from build123d import *

# Parameters (mm, degrees)
ESQUISSE1_R        = 0.068980455
ESQUISSE1_R_2      = 0.06150295
ESQUISSE1_W        = 0.337022694
ESQUISSE1_H        = 5.280022209
BOSS_EXTRU_1_DEPTH = 0.1


with BuildPart() as part:
    # Esquisse1 → Boss.-Extru.1 (new body)
    with BuildSketch(Plane.XY):
        with BuildLine():
            Line((69.009405392, 230.580792913), (69.009405392, 229.722196339))
            ThreePointArc((69.009405392, 229.722196339), (68.979401433, 229.479075631), (68.891190034, 229.250544089))
            Line((68.891190034, 229.250544089), (68.752437477, 228.991137135))
            ThreePointArc((68.752437477, 228.991137135), (68.664226077, 228.762605593), (68.634222119, 228.519484885))
            Line((68.634222119, 228.519484885), (68.634222119, 222.299593089))
            ThreePointArc((68.634222119, 222.299593089), (68.467011491, 221.746003113), (68.021298395, 221.377545392))
            Line((68.021298395, 221.377545392), (63.492336438, 219.476283954))
            ThreePointArc((63.492336438, 219.476283954), (63.046623342, 219.107826233), (62.879412715, 218.554236256))
            Line((62.879412715, 218.554236256), (62.879412715, 215.999425613))
            ThreePointArc((62.879412715, 215.999425613), (62.823397918, 215.841724183), (62.680454788, 215.754691662))
            ThreePointArc((62.680454788, 215.754691662), (62.265082422, 215.243750871), (62.680454788, 214.732810081))
            ThreePointArc((62.680454788, 214.732810081), (62.823397918, 214.645777559), (62.879412715, 214.48807613))
            Line((62.879412715, 214.48807613), (62.879412715, 211.933337892))
            ThreePointArc((62.879412715, 211.933337892), (62.80618941, 211.756561196), (62.629412715, 211.683337892))
            Line((62.629412715, 211.683337892), (50.34681626, 211.683337892))
            ThreePointArc((50.34681626, 211.683337892), (50.170039564, 211.756561196), (50.09681626, 211.933337892))
            Line((50.09681626, 211.933337892), (50.09681626, 214.506095719))
            ThreePointArc((50.09681626, 214.506095719), (50.14774452, 214.657325486), (50.2797798, 214.746940302))
            ThreePointArc((50.2797798, 214.746940302), (50.65644704, 215.242767306), (50.2797798, 215.73859431))
            ThreePointArc((50.2797798, 215.73859431), (50.14774452, 215.828209125), (50.09681626, 215.979438893))
            Line((50.09681626, 215.979438893), (50.09681626, 217.526780439))
            ThreePointArc((50.09681626, 217.526780439), (49.803923041, 218.233887221), (49.09681626, 218.526780439))
            Line((49.09681626, 218.526780439), (43.115034211, 218.526780439))
            ThreePointArc((43.115034211, 218.526780439), (42.40792743, 218.819673658), (42.115034211, 219.526780439))
            Line((42.115034211, 219.526780439), (42.115034211, 223.236736654))
            ThreePointArc((42.115034211, 223.236736654), (42.40792743, 223.943843435), (43.115034211, 224.236736654))
            Line((43.115034211, 224.236736654), (44.704420557, 224.236736654))
            ThreePointArc((44.704420557, 224.236736654), (44.881197252, 224.309959959), (44.954420557, 224.486736654))
            Line((44.954420557, 224.486736654), (44.954420557, 230.580792913))
            Line((44.954420557, 230.580792913), (69.009405392, 230.580792913))
        make_face()
        with Locations((50.977150622, 213.618363216)):
            Circle(ESQUISSE1_R, mode=Mode.SUBTRACT)
        with Locations((61.924613366, 213.618363216)):
            Circle(ESQUISSE1_R_2, mode=Mode.SUBTRACT)
        with Locations((47.409826256, 227.722685683)):
            Rectangle(ESQUISSE1_W, ESQUISSE1_H, mode=Mode.SUBTRACT)
    extrude(amount=BOSS_EXTRU_1_DEPTH)


solid = part.part
Here's how the part is built. I have some questions about the finished solid (model axes, mm). Round coordinates to 2 decimals unless told otherwise and drop trailing zeros. Loops run counter-clockwise (first coordinate to the right, second up) from the corner with the lowest first, then second, coordinate; pieces in that order, holes last. Notation, with made-up numbers: M 16,61 L 51,61 A19 cw 51,76 Z; hole C -12,59 d1. An arc over 180 degrees is marked long. Write each question's results on one line, items separated by ' | '. Start each with the question number.
(1) If I drill on probe 1 along Y at (x, z) = (50.5, 0.05); probe 2 along X at (y, z) = (214, 0.05); probe 3 along Y at (x, z) = (44.25, 0.05), over which ranges is the centre line in solid material (lowest first)? Write a range as from..to.
(2) I want a section at B-B (x = 48.5). Please give me the cut outline in (y, z), then the cut area to 3 significant figures.
(3) I want a section at A-A (y = 226). Please give me the cut outline in (x, z), then the cut area to 3 significant figures.
(4) I want a section at C-C (y = 219). Please give me the cut outline in (x, z), then the cut area to 3 significant figures.
(5) Will this pin go through, and if not, where does the flat tip stop? P1, Ø8, axis at x = 53, y = 226, coming from the -Z side.
Solved:
1) probe 1: y = 211.68..214.87, 215.61..230.58 | probe 2: x = 50.1..62.88 | probe 3: y = 218.53..224.24
2) outline: M 218.53,0 L 230.58,0 L 230.58,0.1 L 218.53,0.1 Z | area: 1.21 mm²
3) outline: M 44.95,0 L 47.24,0 L 47.24,0.1 L 44.95,0.1 Z; M 47.58,0 L 68.63,0 L 68.63,0.1 L 47.58,0.1 Z | area: 2.33 mm²
4) outline: M 42.27,0 L 62.98,0 L 62.98,0.1 L 42.27,0.1 Z | area: 2.07 mm²
5) P1: stops at z = 0
